```python
from build123d import *


with BuildPart() as f2:
    # F2: sweep along a path in F0
    with BuildLine(Plane.XY) as f2_path:
        Line((-325, 150), (-325, -150))
        Line((-325, -150), (325, -150))
        Line((325, -150), (325, 150))
        Line((325, 150), (-325, 150))
    # F1 (on Right) → F2 (sweep)
    with BuildSketch(Plane.YZ):
        with BuildLine():
            Line((125, -70), (131.3123023267, -70))
            Line((131.3123023267, -70), (150, -70))
            Line((150, -70), (150, -66))
            Line((150, -66), (133.8930228842, -66))
            ThreePointArc((133.8930228842, -66), (152.6576287858, 0), (133.8930228842, 66))
            Line((133.8930228842, 66), (150, 66))
            Line((150, 66), (150, 70))
            Line((150, 70), (131.3123023267, 70))
            Line((131.3123023267, 70), (125, 70))
            ThreePointArc((125, 70), (144.0386823701, 0), (125, -70))
        make_face()
    sweep(path=f2_path.line, transition=Transition.RIGHT)


solid = f2.part
```
Check sheet for the modelled part. Datum: model origin and axes. Units: mm. A direction names the side the tool comes from. Round coordinates to 2 decimals unless told otherwise and drop trailing zeros. Order: outer loops, then holes, each group sorted by start corner. A loop starts at its lowest first (then second) coordinate and runs counter-clockwise, first axis right, second up.
1) Section check A-A (x = 36). Record the boundary of the cut face in (y, z).
2) Tool access check on faces 3 (the flat face through (-26, 133, 70)), 4 (the cylindrical face through (-319.035, -2.017, 1.028)). Record the directions out of +Z, -Z, +X, -X, +Y, -Y that give a thin tool (end or side, any length) a straight path to the whole face; none if there is none.
3) Scan lines: line 1 (Y direction, x = -215.5, z = -3.5); line 2 (Z direction, x = 270.5, y = -127); line 3 (Y direction, x = -149.5, z = -26). Record each from-to range of solid material in increasing order.
4) Section check C-C (z = -44). Record the boundary of the cut face in (x, y).
5) Section check D-D (z = 23.5). Record the boundary of the cut face in (x, y).
6) Section check B-B (y = 59). Record the boundary of the cut face in (x, z).
7) Mould release check, pull along X, two halves, no side actions. Record for faces 1 (the flat face through (26, 133, -70)), 2 (the cylindrical face through (4.467, -144.035, 1.028)): +X half, -X half, draft (parallel to the pull), parting line (faces both ways), or undercut.
8) Go/stop test with flat-tipped pins: pin 1 Ø3 at (y, z) = (-21.5, -68.5) entering from +X; pin 2 Ø12 at (y, z) = (-10.5, -13.5) entering from -X; pin 3 Ø1 at (x, z) = (-166, 17.5) entering from -Y. Record where each tip stops, or that it passes through.
Result:
1. outline: (-150, -70) - (-125, -70) arc R138.2 cw to (-125, 70) - (-150, 70) - (-150, 66) - (-133.89, 66) arc R125.45 ccw to (-133.89, -66) - (-150, -66) - close; (125, -70) - (150, -70) - (150, -66) - (133.89, -66) arc R125.45 ccw to (133.89, 66) - (150, 66) - (150, 70) - (125, 70) arc R138.2 cw to start
2. face 3: +Z, +X, -X, +Y, -Y
2. face 4: none
3. line 1: y = -152.61 to -143.99, 143.99 to 152.61
3. line 2: z = -70 to -66.48, 66.48 to 70
3. line 3: y = -149.93 to -141.57, 141.57 to 149.93
4. outline: (-319.69, -144.69) - (319.69, -144.69) - (319.69, 144.69) - (-319.69, 144.69) - close; hole (-311.85, -136.85) - (311.85, -136.85) - (311.85, 136.85) - (-311.85, 136.85) - close
5. outline: (-325.44, -150.44) - (325.44, -150.44) - (325.44, 150.44) - (-325.44, 150.44) - close; hole (-317.03, -142.03) - (317.03, -142.03) - (317.03, 142.03) - (-317.03, 142.03) - close
6. outline: (-325, -70) - (-300, -70) arc R138.2 cw to (-300, 70) - (-325, 70) - (-325, 66) - (-308.89, 66) arc R125.45 ccw to (-308.89, -66) - (-325, -66) - close; (300, -70) - (325, -70) - (325, -66) - (308.89, -66) arc R125.45 ccw to (308.89, 66) - (325, 66) - (325, 70) - (300, 70) arc R138.2 cw to start
7. face 1: draft
7. face 2: undercut
8. pin 1: stops at x = 325
8. pin 2: stops at x = -327.43
8. pin 3: stops at y = -151.5
